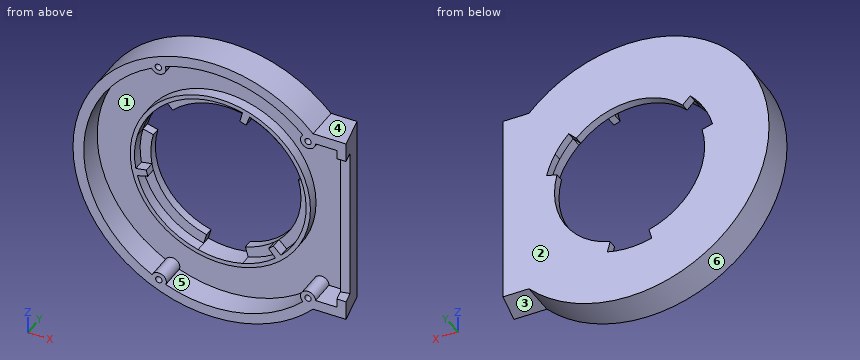
```python
from build123d import *

# Parameters (mm, degrees)
BOSS_EXTRUDE1_DEPTH = 16
CUT_EXTRUDE1_DEPTH  = 12
SKETCH4_W           = 72
SKETCH4_H           = 5
CUT_EXTRUDE2_DEPTH  = 16
SKETCH5_R           = 35
CUT_EXTRUDE3_DEPTH  = 16
CUT_EXTRUDE4_DEPTH  = 10
SKETCH7_R           = 42
BOSS_EXTRUDE2_DEPTH = 5
SKETCH8_R           = 3.5
SKETCH8_R_2         = 1.5
BOSS_EXTRUDE3_DEPTH = 12
SKETCH13_R          = 1.5
CUT_EXTRUDE5_DEPTH  = 12
SKETCH15_W          = 14.23560612
SKETCH15_H          = 16
BOSS_EXTRUDE4_DEPTH = 90
CUT_EXTRUDE6_DEPTH  = 90
CUT_EXTRUDE11_START = -4.8
CUT_EXTRUDE11_DEPTH = 80.4
SKETCH19_W          = 72
SKETCH19_H          = 6
CUT_EXTRUDE14_DEPTH = 8.4


with BuildPart() as part:
    # Sketch1 → Boss-Extrude1 (new body)
    with BuildSketch(Plane(origin=(0, 0, 0), x_dir=(1, 0, 0), z_dir=(0, 1, 0))):
        with BuildLine():
            Line((25, -45.0001724), (25, 44.9998276))
            Line((25, 44.9998276), (46.904322999, 44.9998276))
            ThreePointArc((46.904322999, 44.9998276), (-65, 0.000238913), (46.903992196, -45.0001724))
            Line((46.903992196, -45.0001724), (25, -45.0001724))
        make_face()
        with BuildLine():
            Line((46.904322999, 44.9998276), (25, 44.9998276))
            Line((25, 44.9998276), (25, -45.0001724))
            Line((25, -45.0001724), (46.903992196, -45.0001724))
            ThreePointArc((46.903992196, -45.0001724), (60.306548122, -24.251190767), (65, 0))
            ThreePointArc((65, 0), (60.306637259, 24.250969105), (46.904322999, 44.9998276))
        make_face()
        with BuildLine():
            Line((69, 44.9998276), (46.904322999, 44.9998276))
            ThreePointArc((46.904322999, 44.9998276), (60.306637259, 24.250969105), (65, 0))
            ThreePointArc((65, 0), (60.306548122, -24.251190767), (46.903992196, -45.0001724))
            Line((46.903992196, -45.0001724), (69, -45.0001724))
            Line((69, -45.0001724), (69, 44.9998276))
        make_face()
    extrude(amount=BOSS_EXTRUDE1_DEPTH)

    # Sketch3 → Cut-Extrude1 (cut)
    with BuildSketch(Plane.XZ):
        with BuildLine():
            Line((13.648760289, 40.2001724), (44.541510291, 40.2001724))
            ThreePointArc((44.541510291, 40.2001724), (-60, -0.000232232), (44.541821482, -40.1998276))
            Line((44.541821482, -40.1998276), (13.648760289, -40.1998276))
            Line((13.648760289, -40.1998276), (13.648760289, 40.2001724))
        make_face()
        with BuildLine():
            ThreePointArc((60, 0), (56.002190214, 21.53496439), (44.541510291, 40.2001724))
            Line((44.541510291, 40.2001724), (13.648760289, 40.2001724))
            Line((13.648760289, 40.2001724), (13.648760289, -40.1998276))
            Line((13.648760289, -40.1998276), (44.541821482, -40.1998276))
            ThreePointArc((44.541821482, -40.1998276), (56.002273565, -21.534747631), (60, 0))
        make_face()
        with BuildLine():
            Line((64, -40.1998276), (64, 40.2001724))
            Line((64, 40.2001724), (44.541510291, 40.2001724))
            ThreePointArc((44.541510291, 40.2001724), (56.002190214, 21.53496439), (60, 0))
            ThreePointArc((60, 0), (56.002273565, -21.534747631), (44.541821482, -40.1998276))
            Line((44.541821482, -40.1998276), (64, -40.1998276))
        make_face()
    extrude(amount=-CUT_EXTRUDE1_DEPTH, mode=Mode.SUBTRACT)

    # Sketch4 → Cut-Extrude2 (cut)
    with BuildSketch(Plane(origin=(69, 0, 0), x_dir=(0, 0, -1), z_dir=(1, 0, 0))):
        with Locations((-0.0001724, 2.5)):
            Rectangle(SKETCH4_W, SKETCH4_H)
    extrude(amount=-CUT_EXTRUDE2_DEPTH, mode=Mode.SUBTRACT)

    # Sketch5 → Cut-Extrude3 (cut)
    with BuildSketch(Plane(origin=(0, 16, 0), x_dir=(1, 0, 0), z_dir=(0, 1, 0))):
        Circle(SKETCH5_R)
    extrude(amount=-CUT_EXTRUDE3_DEPTH, mode=Mode.SUBTRACT)

    # Sketch6 → Cut-Extrude4 (cut)
    with BuildSketch(Plane(origin=(0, 16, 0), x_dir=(1, 0, 0), z_dir=(0, 1, 0))):
        with BuildLine():
            Line((-28.284271247, -28.284271247), (-24.748737342, -24.748737342))
            ThreePointArc((-24.748737342, -24.748737342), (-27.76736691, -21.306650015), (-30.310889132, -17.5))
            Line((-30.310889132, -17.5), (-34.641016151, -20))
            ThreePointArc((-34.641016151, -20), (-31.734133612, -24.35045716), (-28.284271247, -28.284271247))
        make_face()
        with BuildLine():
            Line((-34.641016151, -20), (-30.310889132, -17.5))
            ThreePointArc((-30.310889132, -17.5), (-32.335783638, -13.393920133), (-33.80740392, -9.058666579))
            Line((-33.80740392, -9.058666579), (-38.637033052, -10.352761804))
            ThreePointArc((-38.637033052, -10.352761804), (-36.9551813, -15.307337295), (-34.641016151, -20))
        make_face()
        with BuildLine():
            Line((-10.352761804, 38.637033052), (-9.058666579, 33.80740392))
            ThreePointArc((-9.058666579, 33.80740392), (0, 35), (9.058666579, 33.80740392))
            Line((9.058666579, 33.80740392), (10.352761804, 38.637033052))
            ThreePointArc((10.352761804, 38.637033052), (0, 40), (-10.352761804, 38.637033052))
        make_face()
        with BuildLine():
            ThreePointArc((33.831018509, -8.970071717), (32.370760151, -13.309165535), (30.356629112, -17.420535841))
            Line((30.356629112, -17.420535841), (34.693290413, -19.909183818))
            ThreePointArc((34.693290413, -19.909183818), (36.995154458, -15.210474897), (38.664021154, -10.251510534))
            Line((38.664021154, -10.251510534), (33.831018509, -8.970071717))
        make_face()
        with BuildLine():
            ThreePointArc((30.356629112, -17.420535841), (27.823087732, -21.233835948), (24.813485607, -24.683819236))
            Line((24.813485607, -24.683819236), (28.358269265, -28.210079126))
            ThreePointArc((28.358269265, -28.210079126), (31.79781455, -24.267241084), (34.693290413, -19.909183818))
            Line((34.693290413, -19.909183818), (30.356629112, -17.420535841))
        make_face()
    extrude(amount=-CUT_EXTRUDE4_DEPTH, mode=Mode.SUBTRACT)

    # Sketch7 → Boss-Extrude2 (add)
    with BuildSketch(Plane.XZ.offset(-12)):
        Circle(SKETCH7_R)
        with BuildLine():
            ThreePointArc((-28.284271247, 28.284271247), (-10.352761804, 38.637033052), (10.352761804, 38.637033052))
            Line((10.352761804, 38.637033052), (9.058666579, 33.80740392))
            ThreePointArc((9.058666579, 33.80740392), (10.524702983, 33.380093276), (11.970705016, 32.889241728))
            Line((11.970705016, 32.889241728), (13.680805733, 37.587704831))
            ThreePointArc((13.680805733, 37.587704831), (21.53615385, 33.707478063), (28.358269265, 28.210079126))
            ThreePointArc((28.358269265, 28.210079126), (34.693290413, 19.909183818), (38.664021154, 10.251510534))
            ThreePointArc((38.664021154, 10.251510534), (38.623439557, -10.40336084), (28.284271247, -28.284271247))
            Line((28.284271247, -28.284271247), (24.748737342, -24.748737342))
            ThreePointArc((24.748737342, -24.748737342), (23.645657267, -25.804706788), (22.497566339, -26.811555509))
            Line((22.497566339, -26.811555509), (25.711504387, -30.641777725))
            ThreePointArc((25.711504387, -30.641777725), (18.469944529, -35.480433327), (10.352761804, -38.637033052))
            ThreePointArc((10.352761804, -38.637033052), (0, -40), (-10.352761804, -38.637033052))
            ThreePointArc((-10.352761804, -38.637033052), (-28.284271247, -28.284271247), (-38.637033052, -10.352761804))
            Line((-38.637033052, -10.352761804), (-33.80740392, -9.058666579))
            ThreePointArc((-33.80740392, -9.058666579), (-34.170360249, -7.575386488), (-34.468271355, -6.077686218))
            Line((-34.468271355, -6.077686218), (-39.39231012, -6.945927107))
            ThreePointArc((-39.39231012, -6.945927107), (-39.961928863, 1.744775495), (-38.637033052, 10.352761804))
            ThreePointArc((-38.637033052, 10.352761804), (-34.641016151, 20), (-28.284271247, 28.284271247))
        make_face(mode=Mode.SUBTRACT)
    extrude(amount=BOSS_EXTRUDE2_DEPTH)

    # Sketch8 → Boss-Extrude3 (add)
    with BuildSketch(Plane.XZ.offset(-12)):
        with Locations((-25.212285918, 54.445758685)):
            Circle(SKETCH8_R)
        with Locations((-25.212285918, 54.445758685)):
            Circle(SKETCH8_R_2, mode=Mode.SUBTRACT)
        with Locations((-25, -54.543560573)):
            Circle(SKETCH8_R)
        with Locations((-25, -54.543560573)):
            Circle(SKETCH8_R_2, mode=Mode.SUBTRACT)
        with Locations((44.541510291, 40.2001724)):
            Circle(SKETCH8_R)
        with Locations((44.541510291, 40.2001724)):
            Circle(SKETCH8_R_2, mode=Mode.SUBTRACT)
        with Locations((44.541821482, -40.1998276)):
            Circle(SKETCH8_R)
        with Locations((44.541821482, -40.1998276)):
            Circle(SKETCH8_R_2, mode=Mode.SUBTRACT)
    extrude(amount=BOSS_EXTRUDE3_DEPTH)

    # Sketch13 → Cut-Extrude5 (cut)
    with BuildSketch(Plane.XZ.offset(-12)):
        with Locations((44.541510291, 40.2001724)):
            Circle(SKETCH13_R)
        with Locations((-25.212285918, 54.445758685)):
            Circle(SKETCH13_R)
        with Locations((-25, -54.543560573)):
            Circle(SKETCH13_R)
        with Locations((44.541821482, -40.1998276)):
            Circle(SKETCH13_R)
    extrude(amount=CUT_EXTRUDE5_DEPTH, mode=Mode.SUBTRACT)

    # Sketch15 → Boss-Extrude4 (add)
    with BuildSketch(Plane.XY.offset(45.0001724)):
        with Locations((61.88219694, 8)):
            Rectangle(SKETCH15_W, SKETCH15_H)
    extrude(amount=-BOSS_EXTRUDE4_DEPTH)

    # Sketch14 → Cut-Extrude6 (cut)
    with BuildSketch(Plane(origin=(0, 0, -44.9998276), x_dir=(-1, 0, 0), z_dir=(0, 0, -1))):
        Polygon((-69, 16), (-59, 16), (-69, -33), align=None)
    extrude(amount=-CUT_EXTRUDE6_DEPTH, mode=Mode.SUBTRACT)

    # Sketch17 → Cut-Extrude11 (cut)
    with BuildSketch(Plane.XY.offset(45.0001724).offset(CUT_EXTRUDE11_START)):
        Polygon((58.000000002, 0), (54.73469388, 0), (54.73469388, 12), (55.551020411, 12), align=None)
    extrude(amount=-CUT_EXTRUDE11_DEPTH, mode=Mode.SUBTRACT)

    # Sketch19 → Cut-Extrude14 (cut)
    with BuildSketch(Plane(origin=(59.775689724, 12.199120352, 0), x_dir=(0, 0, -1), z_dir=(0.979804059, 0.199960012, 0))):
        with Locations((-0.0001724, -9.450571359)):
            Rectangle(SKETCH19_W, SKETCH19_H)
    extrude(amount=-CUT_EXTRUDE14_DEPTH, mode=Mode.SUBTRACT)


solid = part.part
```
For this review, take the finished solid that the model builds, in its own axes (mm). Face numbers are marked on the shaded views. A direction names the side the tool comes from. Give positions to 0.01 mm unless a question says otherwise; leave off trailing zeros. Loops run counter-clockwise (first coordinate to the right, second up) from the corner with the lowest first, then second, coordinate; pieces in that order, holes last. Notation, with made-up numbers: M 43,72 L 76,72 A12 ccw 76,79 Z; hole C 78.5,40.25 d5. An arc over 180 degrees is marked long. One line per item, written item: value. Start each with the question number.
Q1. For L1, parallel to Z at x = -25, y = 2.25; L2, parallel to X at y = 10.5, z = -33; L3, parallel to X at y = 9.5, z = -32, list the stretches that pass through material, from the lowest coordinate up.
Q2. Clearance check with flat-ended pins moving along their axes: pin 1 Ø3 at (y, z) = (8, -7) entering from -X; pin 2 Ø7.5 at (x, y) = (55, 5.5) entering from +Z; pin 3 Ø8 at (x, y) = (51, 9) entering from -Z; pin 4 Ø25 at (x, z) = (-13.5, -14.5) entering from -Y (1 decimal). State where each tip first meets the part, or that it passes through.
Q3. Add section D-D (z = 49). Give the boundary of the cut face in (x, y), and give its area (3 significant figures).
Q4. Add section C-C (y = 3). Give the boundary of the cut face in (x, z).
Q5. Add section B-B (x = 0). Give the boundary of the cut face in (y, z).
Q6. Add section A-A (z = 0). Give the boundary of the cut face in (x, y).
Q7. Draft analysis for pull direction X (two halves, no side actions). For the marked faces 4, 5 and 6, state which applies: released by +X, released by -X, zero draft, split by the parting line, or undercut.
Q8. Machinability: for the marked faces 1, 2 and 3, which of the approach directions +Z, -Z, +X, -X, +Y, -Y give a long, thin tool a straight path to every point of the face, cutting with its end or side? Answer none if there is none.
Reply:
1. L1: -60 to -56.04, -53.04 to -51.04, 50.95 to 52.96, 55.93 to 60
1. L2: -56 to -50.11, -25.98 to -22.61, 22.61 to 25.98, 55.86 to 60.12
1. L3: -56.58 to -50.75, -27.2 to -24, 24 to 27.2, 56.06 to 60.33
2. pin 1: x = -64.77
2. pin 2: z = 45
2. pin 3: z = -45
2. pin 4: through
3. outline: M -42.71,0 L -34.63,0 L -34.63,12 L 34.63,12 L 34.63,0 L 42.71,0 L 42.71,16 L -42.71,16 Z
3. area: 536 mm²
4. outline: M -28.34,52.88 A3.5 ccw -21.99,55.82 A60 cw 42.12,42.73 A3.5 ccw long 48.04,40.2 L 57.39,40.2 L 57.39,36 L 61.65,36 L 61.65,45 L 46.9,45 A65 ccw long 46.9,-45 L 61.65,-45 L 61.65,-36 L 57.39,-36 L 57.39,-40.2 L 48.04,-40.2 A3.5 ccw long 42.12,-42.73 A60 cw -21.78,-55.91 A3.5 ccw -28.14,-52.99 A60 cw Z; hole C -25.21,54.45 d3; hole C -25,-54.54 d3; hole C 44.54,-40.2 d3; hole C 44.54,40.2 d3
5. outline: M 0,-65 L 16,-65 L 16,-40 L 7,-40 L 7,-42 L 12,-42 L 12,-60 L 0,-60 Z; M 0,60 L 12,60 L 12,42 L 7,42 L 7,40 L 12,40 L 12,35 L 16,35 L 16,65 L 0,65 Z
6. outline: M -65,0 L -60,0 L -60,12 L -42,12 L -42,7 L -40,7 L -40,12 L -35,12 L -35,16 L -65,16 Z; M 35,12 L 40,12 L 40,7 L 42,7 L 42,12 L 55.55,12 L 56.97,5.04 L 61.07,5.88 L 59,16 L 35,16 Z
7. face 4: zero draft
7. face 5: undercut
7. face 6: split by the parting line
8. face 1: -Y
8. face 2: +Z, -Z, +X, -X, +Y
8. face 3: -Z, +X, +Y, -Y
